```python
from build123d import *

# Parameters (mm, degrees)
SKETCH1_R           = 8.55
SKETCH1_R_2         = 7.55
BOSS_EXTRUDE1_DEPTH = 30
SKETCH2_R           = 8.55
BOSS_EXTRUDE2_DEPTH = 2
BOSS_EXTRUDE3_DEPTH = 2
SKETCH4_W           = 2
SKETCH4_H           = 30
BOSS_EXTRUDE4_DEPTH = 5
SKETCH6_W           = 30
SKETCH6_H           = 2
BOSS_EXTRUDE5_DEPTH = 3
SKETCH7_W           = 30
SKETCH7_H           = 2
BOSS_EXTRUDE6_DEPTH = 3
CHAMFER1_SIZE       = 3
CHAMFER2_SIZE       = 1
CHAMFER3_SIZE       = 1


with BuildPart() as part:
    # Sketch1 → Boss-Extrude1 (new body)
    with BuildSketch(Plane(origin=(0, 0, 0), x_dir=(1, 0, 0), z_dir=(0, 1, 0))):
        Circle(SKETCH1_R)
        Circle(SKETCH1_R_2, mode=Mode.SUBTRACT)
    extrude(amount=BOSS_EXTRUDE1_DEPTH)

    # Sketch2 → Boss-Extrude2 (add)
    with BuildSketch(Plane(origin=(0, 30, 0), x_dir=(1, 0, 0), z_dir=(0, 1, 0))):
        Circle(SKETCH2_R)
    extrude(amount=-BOSS_EXTRUDE2_DEPTH)

    # Sketch3 → Boss-Extrude3 (add)
    with BuildSketch(Plane(origin=(0, 30, 0), x_dir=(1, 0, 0), z_dir=(0, 1, 0))):
        Polygon((27.1, -15), (27.1, 15), (25, 15), (-25, 15), (-27.1, 15), (-27.1, -15), (-25, -15), (25, -15), align=None)
    extrude(amount=BOSS_EXTRUDE3_DEPTH)

    # Sketch4 → Boss-Extrude4 (add)
    with BuildSketch(Plane(origin=(0, 32, 0), x_dir=(1, 0, 0), z_dir=(0, 1, 0))):
        with Locations((-26.1, 0)):
            Rectangle(SKETCH4_W, SKETCH4_H)
        with Locations((26.1, 0)):
            Rectangle(SKETCH4_W, SKETCH4_H)
    extrude(amount=BOSS_EXTRUDE4_DEPTH)

    # Sketch6 → Boss-Extrude5 (add)
    with BuildSketch(Plane(origin=(-25.1, 0, 0), x_dir=(0, 0, -1), z_dir=(1, 0, 0))):
        with Locations((0, 36)):
            Rectangle(SKETCH6_W, SKETCH6_H)
    extrude(amount=BOSS_EXTRUDE5_DEPTH)

    # Sketch7 → Boss-Extrude6 (add)
    with BuildSketch(Plane.ZY.offset(-25.1)):
        with Locations((0, 36)):
            Rectangle(SKETCH7_W, SKETCH7_H)
    extrude(amount=BOSS_EXTRUDE6_DEPTH)

    # Chamfer1
    chamfer1_edges = [part.edges().sort_by_distance(p)[0] for p in [
        (-8.55, 30, 0),
    ]]
    chamfer(chamfer1_edges, length=CHAMFER1_SIZE)

    # Chamfer2
    chamfer2_edges = [part.edges().sort_by_distance(p)[0] for p in [
        (-22.1, 35, 0),
        (22.1, 35, 0),
    ]]
    chamfer(chamfer2_edges, length=CHAMFER2_SIZE)

    # Chamfer3
    chamfer3_edges = [part.edges().sort_by_distance(p)[0] for p in [
        (0, 30, -15),
        (27.1, 33.5, -15),
        (-27.1, 30, 0),
        (-27.1, 33.5, -15),
        (0, 30, 15),
        (-27.1, 33.5, 15),
        (27.1, 30, 0),
        (27.1, 33.5, 15),
        (-27.1, 37, 0),
        (27.1, 37, 0),
    ]]
    chamfer(chamfer3_edges, length=CHAMFER3_SIZE)


solid = part.part
```
The listing builds one solid part. Answer for the finished solid, in the listing's coordinates (mm). A direction names the side the tool comes from. Round coordinates to 2 decimals unless told otherwise and drop trailing zeros. Loops run counter-clockwise (first coordinate to the right, second up) from the corner with the lowest first, then second, coordinate; pieces in that order, holes last.
1) A cutting plane is placed at A-A on x = 0. Determine the outline of the cut face in (y, z), plus the area to 3 significant figures.
Outcome:
outline: (0, -8.55) - (27, -8.55) - (30, -11.55) - (30, -14) - (31, -15) - (32, -15) - (32, 15) - (31, 15) - (30, 14) - (30, 11.55) - (27, 8.55) - (0, 8.55) - (0, 7.55) - (28, 7.55) - (28, -7.55) - (0, -7.55) - close
area: 158 mm2
2) Given P1, Ø0.5, axis at y = 36.5, z = -6.5, coming from the -X side; P2, Ø1.6, axis at x = -24, z = -3.5, coming from the -Y side; P3, Ø3, axis at x = -2.5, y = 25.5, coming from the +Z side; P4, Ø12, axis at x = -16, y = 18, coming from the +Z side, each flat-ended and moving along its own axis, determine where each tip first touches the part or whether it passes through.
Outcome:
P1: stops at x = -26.85
P2: stops at y = 30
P3: stops at z = 8.49
P4: passes through
3) For a pull along X with two mould halves and no side action, classify faces 4 (the face through (24, 37, 0)), 5 (the face through (-25.1, 33, 0)), 6 (the face through (0, 28, 0)), 7 (the face through (8.155, 13.311, -2.568)) as released by +X, released by -X, zero draft, split by the parting line, or undercut.
Outcome:
face 4: zero draft
face 5: undercut
face 6: undercut
face 7: split by the parting line
4) A cutting plane is placed at B-B on z = 0. Determine the outline of the cut face in (x, y).
Outcome:
outline: (-27.1, 31) - (-26.1, 30) - (-11.55, 30) - (-8.55, 27) - (-8.55, 0) - (-7.55, 0) - (-7.55, 28) - (7.55, 28) - (7.55, 0) - (8.55, 0) - (8.55, 27) - (11.55, 30) - (26.1, 30) - (27.1, 31) - (27.1, 36) - (26.1, 37) - (22.1, 37) - (22.1, 36) - (23.1, 35) - (25.1, 35) - (25.1, 32) - (-25.1, 32) - (-25.1, 35) - (-23.1, 35) - (-22.1, 36) - (-22.1, 37) - (-26.1, 37) - (-27.1, 36) - close
5) Consider line 1 (Y direction, x = -23.5, z = -12); line 2 (Z direction, x = 0, y = 19). Determine where each line is inside the solid, lowest interval first.
Outcome:
line 1: y = 30 to 32, 35 to 37
line 2: z = -8.55 to -7.55, 7.55 to 8.55
6) A cutting plane is placed at C-C on y = 8.5. Determine the outline of the cut face in (x, z).
Outcome:
outline: circle Ø17.1 at (0, 0); hole circle Ø15.1 at (0, 0)
7) A cutting plane is placed at D-D on x = 13. Determine the outline of the cut face in (y, z).
Outcome:
outline: (30, -14) - (31, -15) - (32, -15) - (32, 15) - (31, 15) - (30, 14) - close
8) For faces 1 (the face through (-1.64, 13.8, 7.37)), 2 (the face through (0, 0, 8)), 3 (the face through (24, 35, 0)), determine the directions among +Z, -Z, +X, -X, +Y, -Y from which every point of the face is accessible in a straight line to the end or side of a thin tool.
Outcome:
face 1: -Y
face 2: +Z, -Z, +X, -X, -Y
face 3: +Z, -Z
